from build123d import *

# Parameters (mm, degrees)
F1_DEPTH = 63.5
F0_W     = 21.5476495911
F0_H     = 19.05
F0_H_2   = 4.74163435
F0_H_3   = 4.78336565
F2_DEPTH = 25.4
F3_DEPTH = 7.9375


with BuildPart() as f1:
    # F0 (on Front) → F1 (new body, symmetric)
    with BuildSketch(Plane.XZ):
        Polygon((2.2602985501, -25.8045658022), (-61.2397014499, -25.8045658022), (-61.2397014499, -44.8545658022), (21.3102985501, -44.8545658022), (21.3102985501, -25.8045658022), align=None)
    extrude(amount=F1_DEPTH, both=True)

    # F0 (on Front) → F2 (join, symmetric)
    with BuildSketch(Plane.XZ):
        with BuildLine():
            Line((2.2602985501, 18.735807389), (2.2602985501, -25.8045658022))
            Line((2.2602985501, -25.8045658022), (21.3102985501, -25.8045658022))
            Line((21.3102985501, -25.8045658022), (21.3102985501, 18.735807389))
            ThreePointArc((21.3102985501, 18.735807389), (24.3886183402, 27.025154163), (32.131285942, 31.2960347603))
            Line((32.131285942, 31.2960347603), (56.6837708669, 31.2960347603))
            Line((56.6837708669, 31.2960347603), (56.6837708669, 50.3460347603))
            Line((56.6837708669, 50.3460347603), (36.9862060647, 50.3460347603))
            ThreePointArc((36.9862060647, 50.3460347603), (12.6376824677, 42.2150276017), (2.2602985501, 18.735807389))
        make_face()
        with Locations((67.4575956625, 40.8210347603)):
            Rectangle(F0_W, F0_H)
        Polygon((107.4837708669, 55.0876691103), (78.231420458, 55.0876691103), (78.231420458, 50.3460347603), (78.231420458, 31.2960347603), (78.231420458, 26.5126691103), (107.4837708669, 26.5126691103), align=None)
        with Locations((67.4575956625, 52.7168519353)):
            Rectangle(F0_W, F0_H_2)
        with Locations((67.4575956625, 28.9043519353)):
            Rectangle(F0_W, F0_H_3)
    extrude(amount=F2_DEPTH, both=True)

    # F0 (on Front) → F3 (join, symmetric)
    with BuildSketch(Plane.XZ):
        with BuildLine():
            add(Edge.make_bspline(
                [(-61.2397014499, -25.8045658022), (-62.6449435949, 22.3603788763), (-18.7473557889, 57.8006356955), (56.6837708669, 55.0876691103)],
                knots=[0, 0, 0, 0, 143.001744718, 143.001744718, 143.001744718, 143.001744718], degree=3))
            Line((-61.2397014499, -25.8045658022), (2.2602985501, -25.8045658022))
            Line((2.2602985501, -25.8045658022), (2.2602985501, 18.735807389))
            ThreePointArc((2.2602985501, 18.735807389), (12.6376824677, 42.2150276017), (36.9862060647, 50.3460347603))
            Line((36.9862060647, 50.3460347603), (56.6837708669, 50.3460347603))
            Line((56.6837708669, 50.3460347603), (56.6837708669, 55.0876691103))
        make_face()
    extrude(amount=F3_DEPTH, both=True)


solid = f1.part
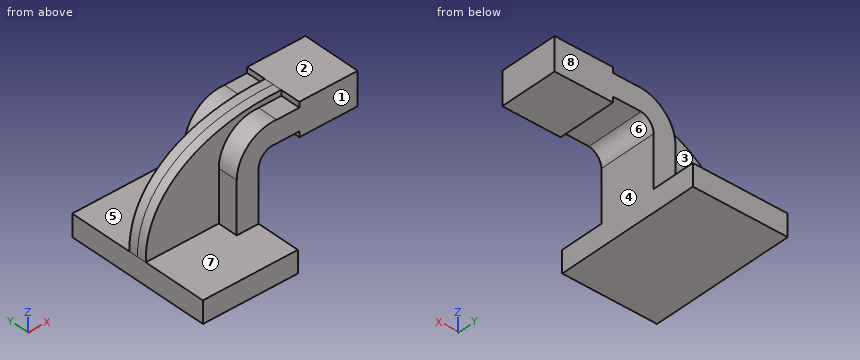
Check sheet for the modelled part. Datum: model origin and axes. Units: mm. Face numbers are marked on the shaded views. A direction names the side the tool comes from. Round coordinates to 2 decimals unless told otherwise and drop trailing zeros. Order: outer loops, then holes, each group sorted by start corner. A loop starts at its lowest first (then second) coordinate and runs counter-clockwise, first axis right, second up. Notation, with made-up numbers: M 47.25,-16 L 98.25,-16 A8 ccw 98.25,-9 Z; hole C 34,52.5 d10. An arc over 180 degrees is marked long. One line per item, written item: value. Start each with the question number.
1. Scan lines: line 1 along X through (y, z) = (-13, -1.5); line 2 along X through (y, z) = (-39.5, -39.5); line 3 along Y through (x, z) = (-14, 10). Record each from-to range of solid material in increasing order.
2. Release check for a two-part mould opening along Y. For the marked faces 1, 2 and 3 record: released by +Y, released by -Y, zero draft, split by the parting line, or undercut.
3. Section check A-A on y = 29. Enter the section's corners in (x, z), and give its area (3 significant figures).
4. Access from +Z, -Z, +X, -X, +Y, -Y to the whole of each face (thin tool, end or side, straight path). Record for the marked faces 4, 5, 6, 7 and 8.
5. Gauge pin test, flat ends, axial feed: P1, Ø7.5, axis at x = 44.5, y = -12, coming from the -Z side; P2, Ø8.5, axis at x = 48.5, y = -17.5, coming from the +Z side; P3, Ø14, axis at y = 16.5, z = 6, coming from the -X side; P4, Ø24.5, axis at x = 51, z = 11, coming from the +Y side. Record the tip position at first contact, or that the pin passes through.
6. Section check B-B on x = 74.5. Enter the section's corners in (y, z).
Results found:
1. line 1: 2.26 to 21.31
1. line 2: -61.24 to 21.31
1. line 3: -7.94 to 7.94
2. face 1: released by -Y
2. face 2: zero draft
2. face 3: released by +Y
3. outline: M -61.24,-44.85 L 21.31,-44.85 L 21.31,-25.8 L -61.24,-25.8 Z
3. area: 1,570 mm^2
4. face 4: -Z, +X, +Y, -Y
4. face 5: +Z, -X, +Y
4. face 6: -Z, +Y, -Y
4. face 7: +Z, -X, -Y
4. face 8: +Z, +X, -X, +Y
5. P1: z = 31.3
5. P2: z = 50.35
5. P3: x = 2.26
5. P4: through
6. outline: M -25.4,26.51 L 25.4,26.51 L 25.4,55.09 L -25.4,55.09 Z
